from build123d import *

# Parameters (mm, degrees)
SKETCH_1_R          = 8
EXTRUDE_1_DEPTH     = 3
SHELL_2_T           = -0.5
SKETCH_2_R          = 3.5
CUT_EXTRUDE_2_DEPTH = 12.704699911


with BuildPart() as part:
    # 草图1 → 拉伸1 (new body)
    with BuildSketch(Plane.XY):
        Circle(SKETCH_1_R)
    extrude(amount=EXTRUDE_1_DEPTH)

    # 抽壳2
    shell_2_openings = [part.faces().sort_by_distance(p)[0] for p in [
        (0, 0, 0),
    ]]
    offset(amount=SHELL_2_T, openings=shell_2_openings, kind=Kind.INTERSECTION)

    # 草图2 → 拉伸2 (cut, through all)
    with BuildSketch(Plane.XY.offset(3)):
        Circle(SKETCH_2_R)
    extrude(amount=-CUT_EXTRUDE_2_DEPTH, mode=Mode.SUBTRACT)


solid = part.part
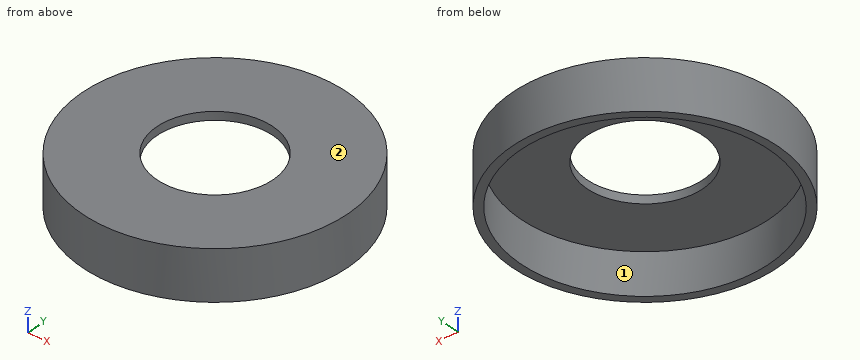
Here's how the part is built. I have some questions about the finished solid (model axes, mm). Face numbers are marked on the shaded views. A direction names the side the tool comes from. Coordinates: 2 decimals unless noted, no trailing zeros. Order: outer loops, then holes, each group sorted by start corner. A loop starts at its lowest first (then second) coordinate and runs counter-clockwise, first axis right, second up. Notation, with made-up numbers: M -10.5,9.25 L 43.5,9.25 A22 cw 43.5,34.25 Z; hole C 82,37 d4. An arc over 180 degrees is marked long. Answer as CSV lines item,"result". Start each with the question number.
1. I want a section at D-D, the plane y = -4. Write out the boundary of the cut face in (x, z).
2. I need wall thicknesses on line 1 (Y direction, x = 0, z = 2.6); line 2 (Z direction, x = -4.75, y = -0.5); line 3 (X direction, y = 0.5, z = 1.6). Which ranges of each line are inside material? Lowest first, please. Write a range as [from, to].
3. For pin 1 (4.5 mm diameter, centred on x = -1, y = -3, fed in from -Z); pin 2 (1.5 mm diameter, centred on y = 4, z = 2, fed in from -X); pin 3 (1.5 mm diameter, centred on y = -2.5, z = 1, fed in from +X); pin 4 (6.5 mm diameter, centred on x = 0, y = 0, fed in from +Z), each with a flat end and sliding along its axis, tell me the tip position at first contact or that it passes through.
4. I want a section at C-C, the plane z = 2.7. Write out the boundary of the cut face in (x, y).
5. I want a section at A-A, the plane y = 0. Write out the boundary of the cut face in (x, z).
6. On a 3-axis mill with a long thin cutter (end or side, diameter ignored), from which of +Z, -Z, +X, -X, +Y, -Y can I reach the whole of each face in a straight line? I mean the marked faces 1 and 2. Say none if no direction works.
Recorded:
1,outline,"M -6.93,0 L -6.34,0 L -6.34,2.5 L 6.34,2.5 L 6.34,0 L 6.93,0 L 6.93,3 L -6.93,3 Z"
2,line 1,"y = [-8, -3.5], [3.5, 8]"
2,line 2,"z = [2.5, 3]"
2,line 3,"x = [-7.98, -7.48], [7.48, 7.98]"
3,pin 1,"stops at z = 2.5"
3,pin 2,"stops at x = -7.31"
3,pin 3,"stops at x = 7.81"
3,pin 4,"passes through"
4,outline,"C 0,0 d16; hole C 0,0 d7"
5,outline,"M -8,0 L -7.5,0 L -7.5,2.5 L -3.5,2.5 L -3.5,3 L -8,3 Z; M 3.5,2.5 L 7.5,2.5 L 7.5,0 L 8,0 L 8,3 L 3.5,3 Z"
6,face 1,"-Z"
6,face 2,"+Z, +X, -X, +Y, -Y"
